Can you work these out from the model? Positions are in its coordinate system, mm. Face numbers are marked on the shaded views. A direction names the side the tool comes from. Give positions to 0.01 mm unless a question says otherwise; leave off trailing zeros. Loops run counter-clockwise (first coordinate to the right, second up) from the corner with the lowest first, then second, coordinate; pieces in that order, holes last. Notation, with made-up numbers: M -29.5,31.5 L 2.5,31.5 A14 ccw 2.5,49.5 Z; hole C 29.5,78.5 d10. An arc over 180 degrees is marked long. Put each result on its own line as item: value. Start each with the question number.
1) Imagine slicing it at B-B (x = 0). Write out the boundary of the cut face in (y, z), then the cut area to 3 significant figures.
2) Please list where these lines run through material, in increasing order: line 1 along Y through (x, z) = (0, -16); line 2 along X through (y, z) = (-49, 13); line 3 along X through (y, z) = (-71, 1). Write a range as from..to.
3) For P1, Ø1.6, axis at x = 37, z = 15.5, coming from the +Y side, with a flat end and sliding along its axis, tell me the tip position at first contact or that it passes through.
4) Imagine slicing it at A-A (x = 69.5). Write out the boundary of the cut face in (y, z), then the cut area to 3 significant figures.
5) Imagine slicing it at D-D (z = 2). State how many separate pieces and enclosed holes the cut face has, then the cut area to 3 significant figures.
6) Imagine slicing it at C-C (y = -16). Write out the boundary of the cut face in (x, z).
7) If we mould it in two halves opening along X, with no side actions, what happens to the marked faces 1, 2 and 3? For each: +X half, -X half, draft (parallel to the pull), parting line (faces both ways), or undercut.
8) For the marked faces 4, 5 and 6, which set-ups out of +Z, -Z, +X, -X, +Y, -Y let a thin tool reach every point of the face, with its end or its side?
from build123d import *

# Parameters (mm, degrees)
CROQUIS1_R              = 36.48
SALIENTE_EXTRUIR1_DEPTH = 35.3


with BuildPart() as part:
    # Croquis1 → Saliente-Extruir1 (new, symmetric)
    with BuildSketch(Plane.XY):
        Polygon((114.170497813, 97.385634303), (103.092241408, 100.742040907), (47.092241408, 100.742040907), (40.383016369, 50.277319492), (-25, 50.277319492), (-105.829502187, 50.277319492), (-105.829502187, -81.012611613), (-74.846281109, -90.399674345), (111.911647615, -90.399674345), (114.170497813, -74.959018563), align=None)
        Circle(CROQUIS1_R, mode=Mode.SUBTRACT)
        with BuildLine():
            Line((39.311090941, -62.873407285), (33.988381842, -62.873407285))
            ThreePointArc((33.988381842, -62.873407285), (33.069143027, -63.25416847), (32.688381842, -64.173407285))
            Line((32.688381842, -64.173407285), (25.899736392, -64.173407285))
            Line((25.899736392, -64.173407285), (25.899736392, -51.012611613))
            Line((25.899736392, -51.012611613), (17.468766423, -51.012611613))
            Line((17.468766423, -51.012611613), (17.468766423, -64.173407285))
            Line((17.468766423, -64.173407285), (17.468766423, -81.012611613))
            Line((17.468766423, -81.012611613), (-71.573973225, -81.012611613))
            Line((-71.573973225, -81.012611613), (-71.573973225, -65.27493481))
            Line((-71.573973225, -65.27493481), (-45.773973225, -65.27493481))
            Line((-45.773973225, -65.27493481), (-45.773973225, -56.101811779))
            Line((-45.773973225, -56.101811779), (-71.573973225, -56.101811779))
            Line((-71.573973225, -56.101811779), (-71.573973225, -40.601811779))
            Line((-71.573973225, -40.601811779), (-43.629552583, -40.601811779))
            Line((-43.629552583, -40.601811779), (-43.629552583, -35.286923245))
            Line((-43.629552583, -35.286923245), (-95.529552548, -35.288826129))
            Line((-95.529552548, -35.288826129), (-95.530450826, -10.788826145))
            Line((-95.530450826, -10.788826145), (-48.440569068, -10.788826145))
            Line((-48.440569068, -10.788826145), (-48.440569068, -6.028234661))
            Line((-48.440569068, -6.028234661), (-92.440569068, -6.028234661))
            ThreePointArc((-92.440569068, -6.028234661), (-95.977129578, -4.562741665), (-97.440568225, -1.025330565))
            Line((-97.440568225, -1.025330565), (-97.440568225, 8.474669435))
            ThreePointArc((-97.440568225, 8.474669435), (-95.977129578, 12.012080534), (-92.440569068, 13.47757353))
            Line((-92.440569068, 13.47757353), (-48.440569068, 13.47757353))
            Line((-48.440569068, 13.47757353), (-43.508684083, 18.277319492))
            Line((-43.508684083, 18.277319492), (-97.808684083, 18.277319492))
            Line((-97.808684083, 18.277319492), (-97.808684083, 44.277319492))
            Line((-97.808684083, 44.277319492), (-25, 44.277319492))
            ThreePointArc((-25, 44.277319492), (-37.368804618, 23.656765735), (-41.676007876, 0))
            ThreePointArc((-41.676007876, 0), (-18.131354261, -37.525239842), (25.899736392, -32.651084015))
            ThreePointArc((25.899736392, -32.651084015), (36.972896923, -17.738767673), (42.48, 0))
            Line((42.48, 0), (54.170497813, 87.932318843))
            ThreePointArc((54.170497813, 87.932318843), (56.165019227, 92.747519492), (60.980219877, 94.742040907))
            Line((60.980219877, 94.742040907), (101.077345244, 94.742040907))
            ThreePointArc((101.077345244, 94.742040907), (106.092961526, 92.664504619), (108.170497813, 87.648888338))
            Line((108.170497813, 87.648888338), (108.170497813, -77.448237029))
            ThreePointArc((108.170497813, -77.448237029), (106.134468962, -82.363645495), (101.219060497, -84.399674345))
            Line((101.219060497, -84.399674345), (61.121935129, -84.399674345))
            ThreePointArc((61.121935129, -84.399674345), (56.206526664, -82.363645495), (54.170497813, -77.448237029))
            Line((54.170497813, -77.448237029), (54.170497813, -32.651084015))
            Line((54.170497813, -32.651084015), (47.399736392, -32.651084015))
            Line((47.399736392, -32.651084015), (47.399736392, -64.173407285))
            Line((47.399736392, -64.173407285), (40.611090941, -64.173407285))
            ThreePointArc((40.611090941, -64.173407285), (40.230329756, -63.25416847), (39.311090941, -62.873407285))
        make_face(mode=Mode.SUBTRACT)
    extrude(amount=SALIENTE_EXTRUIR1_DEPTH, both=True)


solid = part.part
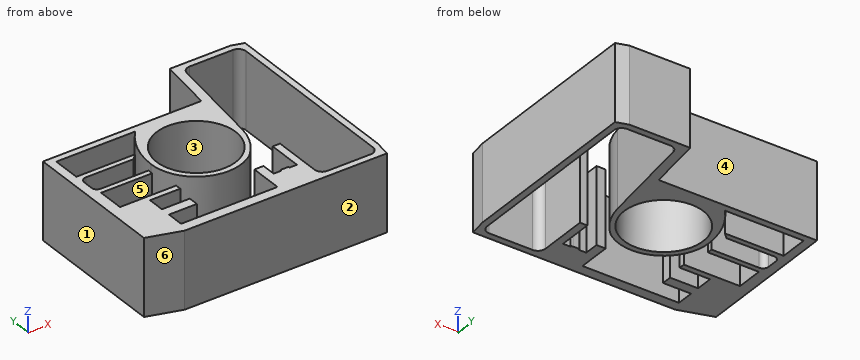
Recorded:
1. outline: M -90.4,-35.3 L -81.01,-35.3 L -81.01,35.3 L -90.4,35.3 Z; M -41.68,-35.3 L -36.48,-35.3 L -36.48,35.3 L -41.68,35.3 Z; M 36.48,-35.3 L 50.28,-35.3 L 50.28,35.3 L 36.48,35.3 Z
1. area: 2,000 mm²
2. line 1: -90.4..-81.01, -41.68..-36.48, 36.48..50.28
2. line 2: -105.83..-71.57, 47.4..54.17, 108.17..114.17
2. line 3: -105.83..-71.57, 17.47..54.17, 108.17..114.17
3. P1: y = 50.28
4. outline: M -90.4,-35.3 L -84.4,-35.3 L -84.4,35.3 L -90.4,35.3 Z; M 94.74,-35.3 L 100.74,-35.3 L 100.74,35.3 L 94.74,35.3 Z
4. area: 847 mm²
5. separate pieces: 1
5. enclosed holes: 2
5. area: 10,800 mm²
6. outline: M -105.83,-35.3 L -95.53,-35.3 L -95.53,35.3 L -105.83,35.3 Z; M -38.48,-35.3 L -32.78,-35.3 L -32.78,35.3 L -38.48,35.3 Z; M 32.78,-35.3 L 37.82,-35.3 L 37.82,35.3 L 32.78,35.3 Z; M 108.17,-35.3 L 114.17,-35.3 L 114.17,35.3 L 108.17,35.3 Z
7. face 1: -X half
7. face 2: draft
7. face 3: undercut
8. face 4: +Z, -Z, -X, +Y
8. face 5: +Z, -Z
8. face 6: +Z, -Z, -X, -Y
